Part model, mm, in its own coordinate system. Face numbers are marked on the shaded views. A direction names the side the tool comes from. Round coordinates to 2 decimals unless told otherwise and drop trailing zeros. Order: outer loops, then holes, each group sorted by start corner. A loop starts at its lowest first (then second) coordinate and runs counter-clockwise, first axis right, second up. Notation, with made-up numbers: (83, 83) - (117, 83) arc R18 cw to (117, 107) - close; hole circle Ø10 at (-32, 60.5). An arc over 180 degrees is marked (long way). Answer as a JSON object with one key per item and string values.
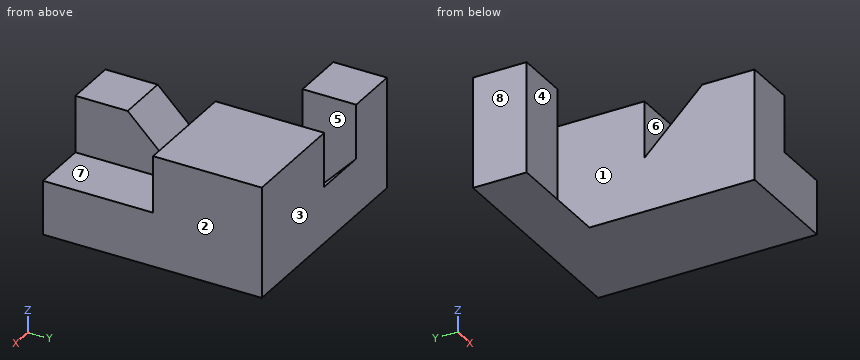
```python
from build123d import *

# Parameters (mm, degrees)
F0_W      = 15.8
F0_H      = 15.8
F1_DEPTH  = 16.1
F3_DEPTH  = 8.1
F5_DEPTH  = 7.8
F6_W      = 15.8
F6_H      = 16
F7_DEPTH  = 7.85
F8_W      = 7.6
F8_H      = 7.6
F9_DEPTH  = 8.25
F11_DEPTH = 7.6
F13_W     = 7.8
F13_H     = 7.8
F14_DEPTH = 25.4


with BuildPart() as f1:
    # F0 (on Top) → F1 (new body)
    with BuildSketch(Plane.XY):
        with Locations((-0.699278047, -1.1891025347)):
            Rectangle(F0_W, F0_H)
    extrude(amount=F1_DEPTH)

    # F2 (on face) → F3 (join)
    with BuildSketch(Plane(origin=(-8.599278047, 0, 0), x_dir=(0, -1, 0), z_dir=(-1, 0, 0))):
        Polygon((1.2891025347, 0), (9.0891025347, 0), (9.0891025347, 8.2), align=None)
    extrude(amount=F3_DEPTH)

    # F4 (on face) → F5 (join)
    with BuildSketch(Plane(origin=(-16.699278047, 0, 0), x_dir=(0, -1, 0), z_dir=(-1, 0, 0))):
        Polygon((1.2891025347, 16.1), (1.2891025347, 0), (9.0891025347, 8.2), (9.0891025347, 16.1), align=None)
        Polygon((1.2891025347, 0), (9.0891025347, 0), (9.0891025347, 8.2), align=None)
    extrude(amount=F5_DEPTH)

    # F6 (on face) → F7 (join)
    with BuildSketch(Plane(origin=(0, 0, 0), x_dir=(1, 0, 0), z_dir=(0, 0, -1))):
        with Locations((-0.699278047, -14.7108974653)):
            Rectangle(F6_W, F6_H)
    extrude(amount=-F7_DEPTH)

    # F8 (on face) → F9 (join, through all)
    with BuildSketch(Plane.XY.offset(7.85)):
        with Locations((-4.799278047, 18.9108974653)):
            Rectangle(F8_W, F8_H)
    extrude(amount=F9_DEPTH)

    # F10 (on face) → F11 (join, through all)
    with BuildSketch(Plane(origin=(-8.599278047, 0, 0), x_dir=(0, -1, 0), z_dir=(-1, 0, 0))):
        Polygon((-6.7108974653, 7.85), (-15.1108974653, 16.1), (-15.1108974653, 7.85), align=None)
    extrude(amount=-F11_DEPTH)

    # F12: F1 across face


with BuildPart() as f1_1:
    add(f1.part)
    add(f1.part.mirror(Plane(origin=(-8.0758652597, -9.0891025347, 7.462251893), x_dir=(1, 0, 0), z_dir=(0, -1, 0))))

    # F13 (on face) → F14 (cut)
    with BuildSketch(Plane.XY.offset(16.1)):
        with Locations((-20.599278047, -5.1891025347)):
            Rectangle(F13_W, F13_H)
        Polygon((-16.699278047, -1.2891025347), (-16.699278047, -9.0891025347), (7.200721953, -9.0891025347), (7.200721953, 22.7108974653), (-24.499278047, 22.7108974653), (-24.499278047, -1.2891025347), align=None)
    extrude(amount=-F14_DEPTH, mode=Mode.SUBTRACT)


solid = f1_1.part
```
Item 1: Cut at D-D (z = 4.5). Write the cut outline in (x, y), plus the area to 3 significant figures.
Taken from the geometry:
{"outline": "(-24.5, -16.89) - (-16.7, -16.89) - (-16.7, -12.61) - (-8.6, -12.61) - (-8.6, -40.89) - (7.2, -40.89) - (7.2, -9.09) - (-24.5, -9.09) - close", "area": "592 mm2"}
Item 2: Two-plate mould, pull along X, no slides. Class the marked faces 1, 2 and 3: pulls with the +X half, pulls with the -X half, needs draft (parallel to the pull), parting line crosses it, or undercut.
Taken from the geometry:
{"face 1": "undercut", "face 2": "pulls with the +X half", "face 3": "needs draft"}
Item 3: Cut at A-A (z = 14.75). Write the cut outline in (x, y), plus the area to 3 significant figures.
Taken from the geometry:
{"outline": "(-24.5, -16.89) - (-16.7, -16.89) - (-16.7, -9.09) - (-24.5, -9.09) - close; (-8.6, -40.89) - (-1, -40.89) - (-1, -31.91) - (-8.6, -31.91) - close; (-8.6, -24.89) - (7.2, -24.89) - (7.2, -9.09) - (-8.6, -9.09) - close", "area": "379 mm2"}
Item 4: Tool access for the marked faces 4, 5, 6, 7 and 8: list every direction of +Z, -Z, +X, -X, +Y, -Y with a clear straight run to the whole face (end or side of a thin tool).
Taken from the geometry:
{"face 4": "+Z, -Z, -X, -Y", "face 5": "+Z, -Y", "face 6": "+Z, +X, -X", "face 7": "+Z, +X, -Y", "face 8": "+Z, -Z, -X, +Y, -Y"}
Item 5: Probe L1, parallel to X at y = -24, z = 15.75; L2, parallel to Z at x = 3.5, y = -31.5; L3, parallel to X at y = -16.5, z = 15.75. List the from-to ranges inside material, lowest first. Write a range as from..to.
Taken from the geometry:
{"L1": "-8.6..7.2", "L2": "0..7.85", "L3": "-24.5..-16.7, -8.6..7.2"}
Item 6: Cut at C-C (y = -14). Write the cut outline in (x, z).
Taken from the geometry:
{"outline": "(-24.5, 0) - (7.2, 0) - (7.2, 16.1) - (-8.6, 16.1) - (-8.6, 3.04) - (-16.7, 3.04) - (-16.7, 16.1) - (-24.5, 16.1) - close"}
Item 7: Cut at B-B (x = -3). Write the cut outline in (y, z), plus the area to 3 significant figures.
Taken from the geometry:
{"outline": "(-40.89, 0) - (-9.09, 0) - (-9.09, 16.1) - (-24.89, 16.1) - (-24.89, 7.85) - (-33.29, 16.1) - (-40.89, 16.1) - close", "area": "477 mm2"}
Item 8: Drop flat-ended pins along their axis: P1, Ø2, axis at x = -15.5, y = -17, coming from the +Z side; P2, Ø1.5, axis at x = -11, y = -23, coming from the -Z side; P3, Ø2.5, axis at x = -22, z = 10, coming from the -Y side; P4, Ø4, axis at x = 1.5, y = -36, coming from the +Z side. Give the stop position or say it passes through.
Taken from the geometry:
{"P1": "z = 0.93", "P2": "through", "P3": "y = -16.89", "P4": "z = 7.85"}
